Verification items for the finished model (mm, model axes). Face numbers are marked on the shaded views. A direction names the side the tool comes from. Round coordinates to 2 decimals unless told otherwise and drop trailing zeros. Order: outer loops, then holes, each group sorted by start corner. A loop starts at its lowest first (then second) coordinate and runs counter-clockwise, first axis right, second up. Notation, with made-up numbers: M 3,-2 L 41,-2 A20 ccw 41,31 Z; hole C 12.5,42.25 d4. An arc over 180 degrees is marked long. Answer as a JSON object with one key per item and string values. Group by question number.
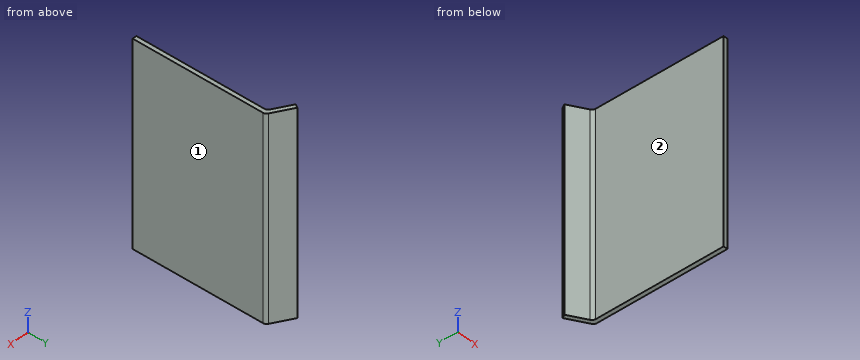
Autodesk Inventor part; units mm, degrees
ref_plane "YZ Plane" through (0, 0, 0) normal (1, 0, 0) x (0, 1, 0)
ref_plane "XZ Plane" through (0, 0, 0) normal (0, 1, 0) x (-1, 0, 0)
ref_plane "XY Plane" through (0, 0, 0) normal (0, 0, 1) x (1, 0, 0)
sketch "Sketch1" plane through (0, 0, 0) normal (0, 0, 1) x (1, 0, 0)
  line L0 (0, 0) -> (6.35, 0)
  line L1 (6.35, 0) -> (6.35, 203.2)
  line L2 (6.35, 203.2) -> (-26.6456, 222.25)
  line L3 (-26.6456, 222.25) -> (-29.8206, 216.7507)
  line L4 (-29.8206, 216.7507) -> (-3.175, 201.3669)
  line L5 (0, 195.8677) -> (0, 0)
  arc A0 (6.35, 199.5338) -> (3.175, 205.0331) centre (0, 199.5338) ccw
  arc A1 (0, 195.8677) -> (-3.175, 201.3669) centre (-6.35, 195.8677) ccw
  dimension "d0" = 6.35
  dimension "d1" = 6.35
  dimension "d2" = 120
  dimension "d3" = 38.1
  dimension "d4" = 203.2
  dimension "d6" = 6.35
extrude "Extrusion1" add sketch "Sketch1" against normal blind 304.8 contours L5 A1 L4 L3 L2 A0 L1 L0
properties part number "GE-13044" material "Polycarbonate, Clear"
Q1. Thickness scan on line 1 (X direction, y = 114.5, z = -161.5); line 2 (Y direction, x = -10, z = -71); line 3 (Y direction, x = -19.5, z = -139.5). Record the ranges inside material, lowest first. Write a range as from..to.
Q2. Cross-section at B-B, the plane y = 170. Record the cut outline in (x, z), then the cut area to 3 significant figures.
Q3. Cross-section at C-C, the plane x = -22. Record the cut outline in (y, z), then the cut area to 3 significant figures.
Q4. Gauge pin test, flat ends, axial feed: pin 1 Ø12 at (y, z) = (80.5, -247.5) entering from -X; pin 2 Ø4 at (x, y) = (-1.5, 180.5) entering from -Z; pin 3 Ø3 at (x, z) = (-5, -44.5) entering from -Y; pin 4 Ø3 at (x, z) = (-9, -164.5) entering from +Y. Record the tip position at first contact, or that the pin passes through.
Q5. Cross-section at A-A, the plane z = -60.5. Record the cut outline in (x, y) (3 decimals).
Q6. Tool access check on the marked faces 1 and 2. Record the directions out of +Z, -Z, +X, -X, +Y, -Y that give a thin tool (end or side, any length) a straight path to the whole face; none if there is none.
Conclusion:
{
 "1": {"line 1": "0..6.35", "line 2": "205.31..212.64", "line 3": "210.79..218.12"},
 "2": {"outline": "M 0,-304.8 L 6.35,-304.8 L 6.35,0 L 0,0 Z", "area": "1,940 mm2"},
 "3": {"outline": "M 212.24,-304.8 L 219.57,-304.8 L 219.57,0 L 212.24,0 Z", "area": "2,230 mm2"},
 "4": {"pin 1": "x = 0", "pin 2": "z = -304.8", "pin 3": "y = 201.55", "pin 4": "y = 212.93"},
 "5": {"outline": "M -29.821,216.751 L -3.175,201.367 A6.35 cw 0,195.868 L 0,0 L 6.35,0 L 6.35,199.534 A6.35 ccw 3.175,205.033 L -26.646,222.25 Z"},
 "6": {"face 1": "+Z, -Z, +X, +Y, -Y", "face 2": "+Z, -Z, -X, -Y"}
}
